```python
from build123d import *

# Parameters (mm, degrees)
SKETCH1_W           = 20
SKETCH1_H           = 25
BOSS_EXTRUDE1_DEPTH = 10
SKETCH3_W           = 2.5
SKETCH3_H           = 9.5
BOSS_EXTRUDE3_DEPTH = 5
SKETCH4_W           = 2.5
SKETCH4_H           = 9.5
BOSS_EXTRUDE4_DEPTH = 5
BOSS_EXTRUDE5_DEPTH = 2.5
SKETCH6_R           = 1.25
BOSS_EXTRUDE6_DEPTH = 3


with BuildPart() as part:
    # Sketch1 → Boss-Extrude1 (new body)
    with BuildSketch(Plane(origin=(0, 0, 0), x_dir=(1, 0, 0), z_dir=(0, 1, 0))):
        Rectangle(SKETCH1_W, SKETCH1_H)
    extrude(amount=BOSS_EXTRUDE1_DEPTH)

    # Sketch3 → Boss-Extrude3 (add)
    with BuildSketch(Plane(origin=(0, 0, -12.5), x_dir=(-1, 0, 0), z_dir=(0, 0, -1))):
        with Locations((-5, 5)):
            Rectangle(SKETCH3_W, SKETCH3_H)
    extrude(amount=BOSS_EXTRUDE3_DEPTH)

    # Sketch4 → Boss-Extrude4 (add)
    with BuildSketch(Plane.XY.offset(12.5)):
        with Locations((5, 5)):
            Rectangle(SKETCH4_W, SKETCH4_H)
    extrude(amount=BOSS_EXTRUDE4_DEPTH)

    # Sketch5 → Boss-Extrude5 (add)
    with BuildSketch(Plane(origin=(10, 0, 0), x_dir=(0, 0, -1), z_dir=(1, 0, 0))):
        with BuildLine():
            ThreePointArc((-2.967408029, 7.110831595), (-12.498528779, 5.121284968), (-3.075116724, 2.671823033))
            ThreePointArc((-3.075116724, 2.671823033), (3.748896584, 4.727055275), (-2.967408029, 7.110831595))
        make_face()
    extrude(amount=BOSS_EXTRUDE5_DEPTH)

    # Sketch6 → Boss-Extrude6 (add)
    with BuildSketch(Plane(origin=(12.5, 0, 0), x_dir=(0, 0, -1), z_dir=(1, 0, 0))):
        with Locations((-7.5, 5)):
            Circle(SKETCH6_R)
    extrude(amount=BOSS_EXTRUDE6_DEPTH)


solid = part.part
```
Read the model definition and answer for the solid it produces. Units are mm, in the model's axes. A direction names the side the tool comes from. Coordinates: 2 decimals unless noted, no trailing zeros. Write each loop counter-clockwise with the first axis right and the second up, starting at its lowest first coordinate (ties: lowest second). Pieces come first, ordered by that corner, then holes. Notation, with made-up numbers: (69, -15) -> (96, -15) arc R24 ccw to (96, 16) -> close; hole circle Ø2 at (27, 25.25). An arc over 180 degrees is marked (long way). Write item = value, one per line.
(1) Section D-D on z = 1 is taken. Write down the section's boundary in (x, y).
From the geometry:
outline = (-10, 0) -> (10, 0) -> (10, 1.2) -> (12.5, 1.2) -> (12.5, 8.43) -> (10, 8.43) -> (10, 10) -> (-10, 10) -> close
(2) Section A-A on x = -0.25 is taken. Write down the section's boundary in (y, z), plus the area to 3 significant figures.
From the geometry:
outline = (0, -12.5) -> (10, -12.5) -> (10, 12.5) -> (0, 12.5) -> close
area = 250 mm2
(3) Straight lines are drawn through the part: L1, parallel to Z at x = 9.5, y = 0.5; L2, parallel to X at y = 0.75, z = 0; L3, parallel to X at y = 8.5, z = -13. For each, find the intervals that lie inside material, in ascending order. Write a range as from..to.
From the geometry:
L1 = -12.5..12.5
L2 = -10..10
L3 = 3.75..6.25
(4) Section C-C on y = 8 is taken. Write down the section's boundary in (x, z).
From the geometry:
outline = (-10, -12.5) -> (3.75, -12.5) -> (3.75, -17.5) -> (6.25, -17.5) -> (6.25, -12.5) -> (10, -12.5) -> (10, -1.98) -> (12.5, -1.98) -> (12.5, 1.98) -> (10, 1.98) -> (10, 3.5) -> (12.5, 3.5) -> (12.5, 11.5) -> (10, 11.5) -> (10, 12.5) -> (6.25, 12.5) -> (6.25, 17.5) -> (3.75, 17.5) -> (3.75, 12.5) -> (-10, 12.5) -> close
(5) Given pin 1 Ø4 at (y, z) = (7.5, 3) entering from +X; pin 2 Ø0.8 at (x, z) = (5.5, -15) entering from +Y; pin 3 Ø1.5 at (y, z) = (3.5, 15) entering from -X, each flat-ended and moving along its own axis, determine where each tip first touches the part or whether it passes through.
From the geometry:
pin_1 = 12.5
pin_2 = 9.75
pin_3 = 3.75
(6) Which of the six approach directions +Z, -Z, +X, -X, +Y, -Y give full straight-line access (tool end or side, diameter ignored) to faces 5 (the face through (5, 0.25, -15)), 6 (the face through (5, 9.75, -15)), 7 (the face through (6.25, 5, 15)), 8 (the face through (6.25, 5, -15)), 9 (the face through (10, 9, 11))?
From the geometry:
face_5 = -Z, +X, -X, -Y
face_6 = -Z, +X, -X, +Y
face_7 = +Z, +X, +Y, -Y
face_8 = -Z, +X, +Y, -Y
face_9 = +Z, +X, +Y
(7) For a pull along Z with two mould halves and no side action, classify faces 1 (the face through (5, 5, 17.5)), 2 (the face through (3.75, 5, 15)), 3 (the face through (5, 5, -17.5)), 4 (the face through (11.232, 4.596, -3.743)) as +Z half, -Z half, draft (parallel to the pull), parting line (faces both ways), or undercut.
From the geometry:
face_1 = +Z half
face_2 = draft
face_3 = -Z half
face_4 = undercut
(8) Section B-B on z = -3 is taken. Write down the section's boundary in (x, y), plus the area to 3 significant figures.
From the geometry:
outline = (-10, 0) -> (10, 0) -> (10, 2.57) -> (12.5, 2.57) -> (12.5, 7.07) -> (10, 7.07) -> (10, 10) -> (-10, 10) -> close
area = 211 mm2
